The model under review builds one solid part; all positions refer to its coordinate system, in mm. Face numbers are marked on the shaded views. A direction names the side the tool comes from. Give positions to 0.01 mm unless a question says otherwise; leave off trailing zeros. Order: outer loops, then holes, each group sorted by start corner. A loop starts at its lowest first (then second) coordinate and runs counter-clockwise, first axis right, second up. Notation, with made-up numbers: (81, -6.5) - (105, -6.5) arc R20 cw to (105, 15.5) - close; hole circle Ø6 at (8.25, 45.25). An arc over 180 degrees is marked (long way). Use CSV: the item, a comma, the result in double quotes.
```python
from build123d import *

# Parameters (mm, degrees)
SKETCH2_W                     = 50.8
SKETCH2_H                     = 71.73468
SKETCH2_W_2                   = 0.9906
SKETCH2_H_2                   = 44.45
BOSS_EXTRUDE1_DEPTH           = 1.5875
SKETCH3_W                     = 50.8
SKETCH3_H                     = 3.175
BOSS_EXTRUDE2_DEPTH           = 6.35
FILLET1_R                     = 3.175
TAP_DRILL_FOR_4_40_TAP1_D     = 2.2606
TAP_DRILL_FOR_4_40_TAP1_DEPTH = 6.35
TAP_DRILL_FOR_4_40_TAP1_TIP   = 0.679152758
SKETCH7_R                     = 3.175
CUT_EXTRUDE1_DEPTH            = 44.45


with BuildPart() as part:
    # Sketch2 → Boss-Extrude1 (new body)
    with BuildSketch(Plane.ZY.offset(-52.8754333)):
        Rectangle(SKETCH2_W, SKETCH2_H)
        Rectangle(SKETCH2_W_2, SKETCH2_H_2, mode=Mode.SUBTRACT)
    extrude(amount=BOSS_EXTRUDE1_DEPTH)

    # Sketch3 → Boss-Extrude2 (add)
    with BuildSketch(Plane.ZY.offset(-52.8754333)):
        with Locations((0, 34.27984)):
            Rectangle(SKETCH3_W, SKETCH3_H)
    extrude(amount=BOSS_EXTRUDE2_DEPTH)

    # Fillet1
    fillet1_edges = [part.edges().sort_by_distance(p)[0] for p in [
        (51.2879333, 32.69234, 0),
    ]]
    fillet(fillet1_edges, radius=FILLET1_R)

    # Tap Drill for #4-40 Tap1
    with Locations(Plane(origin=(0, 35.86734, 0), x_dir=(1, 0, 0), z_dir=(0, 1, 0))):
        with Locations((49.7004333, -22.225), (49.7004333, 22.225)):
            Hole(TAP_DRILL_FOR_4_40_TAP1_D / 2, depth=TAP_DRILL_FOR_4_40_TAP1_DEPTH)
            with Locations((0, 0, -(TAP_DRILL_FOR_4_40_TAP1_DEPTH + TAP_DRILL_FOR_4_40_TAP1_TIP / 2))):  # 118° drill point
                Cone(0, TAP_DRILL_FOR_4_40_TAP1_D / 2, TAP_DRILL_FOR_4_40_TAP1_TIP, mode=Mode.SUBTRACT)

    # Sketch7 → Cut-Extrude1 (cut)
    with BuildSketch(Plane.XZ.offset(-22.225)):
        with Locations((54.42406195, 0)):
            Circle(SKETCH7_R)
    extrude(amount=CUT_EXTRUDE1_DEPTH, mode=Mode.SUBTRACT)


solid = part.part
```
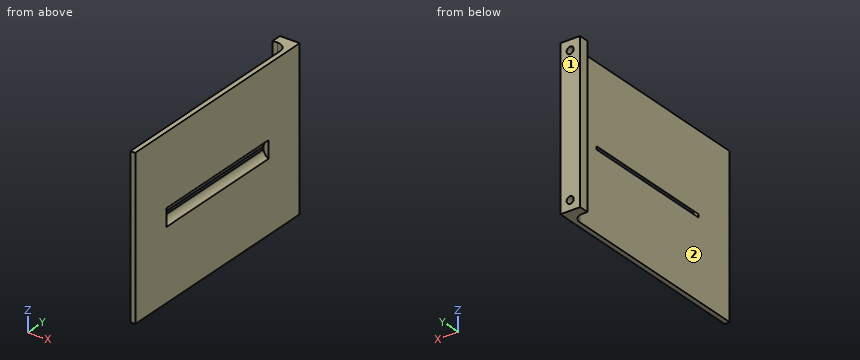
Item 1: Take a section at B-B, the plane z = -15. Give the boundary of the cut face in (x, y) (3 decimals).
Results list:
outline,"(46.525, 32.692) - (48.113, 32.692) arc R3.175 cw to (51.288, 29.517) - (51.288, -35.867) - (52.875, -35.867) - (52.875, 35.867) - (46.525, 35.867) - close"
Item 2: Take a section at A-A, the plane y = 7. Give the boundary of the cut face in (x, z) (3 decimals).
Results list:
outline,"(51.288, -25.4) - (52.875, -25.4) - (52.875, -2.772) arc R3.175 cw to (51.288, -0.495) - close; (51.288, 0.495) arc R3.175 cw to (52.875, 2.772) - (52.875, 25.4) - (51.288, 25.4) - close"
Item 3: Wall thickness on L1, parallel to Y at x = 47.5, z = 3; L2, parallel to X at y = 3, z = 19.5; L3, parallel to Z at x = 52.5, y = 1: over which ranges is each line inside the solid? List them lowest first.
Results list:
L1,"y = 32.69 to 35.87"
L2,"x = 51.29 to 52.88"
L3,"z = -25.4 to -2.53, 2.53 to 25.4"
Item 4: Tool access review of the marked faces 1 and 2: name each direction out of +Z, -Z, +X, -X, +Y, -Y from which nothing blocks a thin tool from reaching the whole face with its end or side.
Results list:
face 1,"+Z, -Z, +X, -X, +Y"
face 2,"+Z, -Z, -X, -Y"
Item 5: Clearance check with flat-ended pins moving along their axes: pin 1 (5 mm diameter, centred on y = 17.5, z = -20, fed in from -X); pin 2 (0.8 mm diameter, centred on x = 47.5, z = -7, fed in from -Y). State where each tip first meets the part, or that it passes through.
Results list:
pin 1,"stops at x = 51.29"
pin 2,"stops at y = 32.69"
Item 6: Take a section at C-C, the plane x = 49.5. Give the boundary of the cut face in (y, z), and give its area (3 significant figures).
Results list:
outline,"(32.37, -25.4) - (35.87, -25.4) - (35.87, -23.34) - (32.37, -23.34) - close; (32.37, -21.11) - (35.87, -21.11) - (35.87, 21.11) - (32.37, 21.11) - close; (32.37, 23.34) - (35.87, 23.34) - (35.87, 25.4) - (32.37, 25.4) - close"
area,"162 mm2"
